Answer from the drawing. Dimensions are ordinates in mm from the lowest x, y and z of the part. Coordinates: 2 decimals unless noted, no trailing zeros. Write each loop counter-clockwise with the first axis right and the second up, starting at its lowest first coordinate (ties: lowest second). Pieces come first, ordered by that corner, then holes.
1) The part is cut by section C-C (z = 7). Determine the outline of the cut face in (x, y) (3 decimals), then the cut area to 3 significant figures.
2) This flat-tipped pin is pushed along its axis until it touches: pin 1 Ø6.5 at (x, z) = (248, 6.5) entering from +Y. Where does it stop, or does it pass through?
3) The part is cut by section B-B (y = 198). Determine the outline of the cut face in (x, z) (3 decimals).
4) Find the intervals of material crossed by line 1 (X direction, y = 200, z = 6) (3 decimals); line 2 (Y direction, x = 63.5, z = 9), in increasing order.
5) The part is cut by section A-A (x = 256). Determine the outline of the cut face in (y, z).
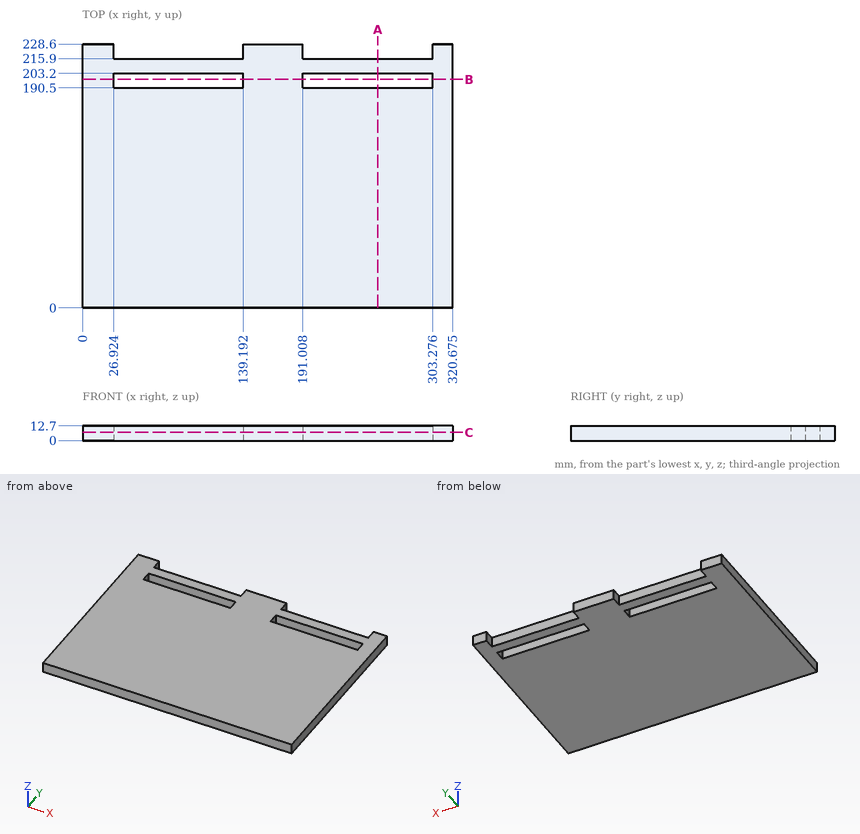
Reported:
1. outline: (0, 0) - (320.675, 0) - (320.675, 228.6) - (303.276, 228.6) - (303.276, 215.9) - (191.008, 215.9) - (191.008, 228.6) - (139.192, 228.6) - (139.192, 215.9) - (26.924, 215.9) - (26.924, 228.6) - (0, 228.6) - close; hole (26.924, 190.5) - (139.192, 190.5) - (139.192, 203.2) - (26.924, 203.2) - close; hole (191.008, 190.5) - (303.276, 190.5) - (303.276, 203.2) - (191.008, 203.2) - close
1. area: 67,600 mm2
2. pin 1: stops at y = 215.9
3. outline: (0, 0) - (26.924, 0) - (26.924, 12.7) - (0, 12.7) - close; (139.192, 0) - (191.008, 0) - (191.008, 12.7) - (139.192, 12.7) - close; (303.276, 0) - (320.675, 0) - (320.675, 12.7) - (303.276, 12.7) - close
4. line 1: x = 0 to 26.924, 139.192 to 191.008, 303.276 to 320.675
4. line 2: y = 0 to 190.5, 203.2 to 215.9
5. outline: (0, 0) - (190.5, 0) - (190.5, 12.7) - (0, 12.7) - close; (203.2, 0) - (215.9, 0) - (215.9, 12.7) - (203.2, 12.7) - close
